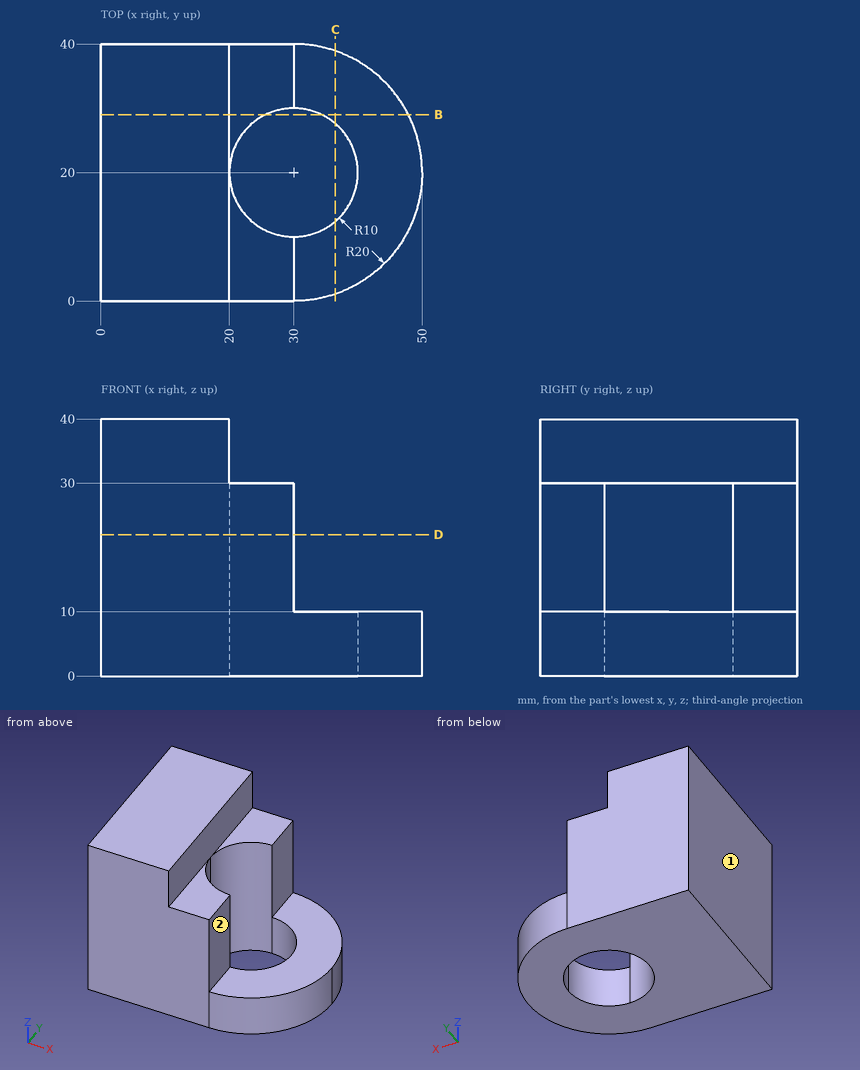
Design review of the part shown in the three views and the two pictorial views. Dimensions are in mm from the part's minimum x, y and z. A direction names the side the tool comes from. Give positions to 0.01 mm unless a question says otherwise; leave off trailing zeros. Loops run counter-clockwise (first coordinate to the right, second up) from the corner with the lowest first, then second, coordinate; pieces in that order, holes last. Notation, with made-up numbers: (50, 69.25) -> (62, 69.25) arc R14 cw to (62, 81.25) -> close; hole circle Ø10 at (77.5, -30.75). An arc over 180 degrees is marked (long way). Answer as a JSON object with one key per item and string values. Group by question number.
Q1. Take a section at B-B (y = 29). Write out the cut boundary in (x, z).
Q2. Wall thickness on line 1 along Z through (x, y) = (28, 31.5); line 2 along X through (y, z) = (21.5, 32.5): over which ranges is each line inside the solid? List them lowest first.
Q3. Take a section at C-C (x = 36.5). Write out the cut boundary in (y, z).
Q4. Take a section at D-D (z = 22). Write out the cut boundary in (x, y).
Q5. Tool access review of the marked faces 1 and 2: name each direction out of +Z, -Z, +X, -X, +Y, -Y from which nothing blocks a thin tool from reaching the whole face with its end or side.
Q6. Insertion check: pin 1 (3 mm diameter, centred on y = 14.5, z = 34, fed in from +X); pin 2 (11 mm diameter, centred on x = 24, y = 13.5, fed in from +Z); pin 3 (10 mm diameter, centred on y = 29, z = 20.5, fed in from +X); pin 4 (3 mm diameter, centred on x = 38.5, y = 5.5, fed in from +Z). Each pin has a flat end and moves straight along its axis. Give the tip position at first contact, or say it passes through.
Answer below:
{
 "1": {"outline": "(0, 0) -> (25.64, 0) -> (25.64, 30) -> (20, 30) -> (20, 40) -> (0, 40) -> close; (34.36, 0) -> (47.86, 0) -> (47.86, 10) -> (34.36, 10) -> close"},
 "2": {"line 1": "z = 0 to 30", "line 2": "x = 0 to 20"},
 "3": {"outline": "(1.09, 0) -> (12.4, 0) -> (12.4, 10) -> (1.09, 10) -> close; (27.6, 0) -> (38.91, 0) -> (38.91, 10) -> (27.6, 10) -> close"},
 "4": {"outline": "(0, 0) -> (30, 0) -> (30, 10) arc R10 cw to (30, 30) -> (30, 40) -> (0, 40) -> close"},
 "5": {"face 1": "+Z, -Z, -X, +Y, -Y", "face 2": "+Z, +X, +Y, -Y"},
 "6": {"pin 1": "stops at x = 20", "pin 2": "stops at z = 40", "pin 3": "stops at x = 30", "pin 4": "stops at z = 10"}
}
